from build123d import *

# Parameters (mm, degrees)
F0_R     = 9
F1_DEPTH = 9
F2_R     = 5
F3_DEPTH = 30
F4_R     = 7.5
F5_DEPTH = 3
F6_R     = 0.5
F7_SIZE  = 0.1


with BuildPart() as f1:
    # F0 (on Top) → F1 (new body)
    with BuildSketch(Plane.XY):
        Circle(F0_R)
    extrude(amount=F1_DEPTH)

    # F2 (on face) → F3 (join)
    with BuildSketch(Plane.XY.offset(9)):
        Circle(F2_R)
    extrude(amount=F3_DEPTH)

    # F4 (on face) → F5 (cut)
    with BuildSketch(Plane(origin=(0, 0, 0), x_dir=(1, 0, 0), z_dir=(0, 0, -1))):
        Circle(F4_R)
    extrude(amount=-F5_DEPTH, mode=Mode.SUBTRACT)

    # F6
    f6_edges = [f1.edges().sort_by_distance(p)[0] for p in [
        (-7.5, 0, 0),
        (-5, 0, 39),
    ]]
    fillet(f6_edges, radius=F6_R)

    # F7
    f7_edges = [f1.edges().sort_by_distance(p)[0] for p in [
        (-9, 0, 9),
    ]]
    chamfer(f7_edges, length=F7_SIZE)


solid = f1.part
The model under review builds one solid part; all positions refer to its coordinate system, in mm. A direction names the side the tool comes from. Coordinates: 2 decimals unless noted, no trailing zeros. Order: outer loops, then holes, each group sorted by start corner. A loop starts at its lowest first (then second) coordinate and runs counter-clockwise, first axis right, second up. Notation, with made-up numbers: (46.25, -11) -> (86.25, -11) arc R29 cw to (86.25, 15) -> close; hole circle Ø4 at (13, -39). An arc over 180 degrees is marked (long way). Answer in a Markdown table with one row per item.
(1) Wall thickness on line 1 along Y through (x, z) = (0, 1.95); line 2 along Z through (x, y) = (-5, 0.75); line 3 along Z through (x, y) = (2.25, 1.75): over which ranges is each line inside the solid? List them lowest first.
Answers:
| item | result |
|---|---|
| line 1 | -9 to -7.5, 7.5 to 9 |
| line 2 | 3 to 9 |
| line 3 | 3 to 39 |
(2) Consider section D-D (z = 4). Write out the cut boundary in (x, y).
Answers:
| item | result |
|---|---|
| outline | circle Ø18 at (0, 0) |
(3) Insertion check: pin 1 (1.5 mm diameter, centred on x = 0.5, z = 10, fed in from +Y); pin 2 (1 mm diameter, centred on x = 1.5, z = 5.5, fed in from -Y); pin 3 (8 mm diameter, centred on y = -5, z = 27.5, fed in from +X). Each pin has a flat end and moves straight along its axis. Give the tip position at first contact, or say it passes through.
Answers:
| item | result |
|---|---|
| pin 1 | y = 5 |
| pin 2 | y = -8.94 |
| pin 3 | x = 4.9 |
(4) The part is to be moulded in two halves that separate along Y. For faces 1 (the flat face through (4, -4, 9)), 2 (the cylindrical face through (-1.08, -4.88, 23.54)), 3 (the flat face through (0, 0, 3)), say which applies: +Y half, -Y half, draft (parallel to the pull), parting line (faces both ways), or undercut.
Answers:
| item | result |
|---|---|
| face 1 | draft |
| face 2 | parting line |
| face 3 | undercut |
(5) Consider section A-A (y = 0). Write out the cut boundary in (x, z).
Answers:
| item | result |
|---|---|
| outline | (-9, 0) -> (-8, 0) arc R0.5 ccw to (-7.5, 0.5) -> (-7.5, 3) -> (7.5, 3) -> (7.5, 0.5) arc R0.5 ccw to (8, 0) -> (9, 0) -> (9, 8.9) -> (8.9, 9) -> (5, 9) -> (5, 38.5) arc R0.5 ccw to (4.5, 39) -> (-4.5, 39) arc R0.5 ccw to (-5, 38.5) -> (-5, 9) -> (-8.9, 9) -> (-9, 8.9) -> close |
(6) Machinability: for faces 4 (the cylindrical face through (-7.493, -0.33, 1.732)), 5 (the flat face through (0, 0, 39)), which of the approach directions +Z, -Z, +X, -X, +Y, -Y give a long, thin tool a straight path to every point of the face, cutting with its end or side? Answer none if there is none.
Answers:
| item | result |
|---|---|
| face 4 | -Z |
| face 5 | +Z, +X, -X, +Y, -Y |
(7) Consider section C-C (z = 26). Write out the cut boundary in (x, y), plus the area to 3 significant figures.
Answers:
| item | result |
|---|---|
| outline | circle Ø10 at (0, 0) |
| area | 78.5 mm² |
